Work out the finished part from the listing and answer in its coordinate system (mm). A direction names the side the tool comes from. Give positions to 0.01 mm unless a question says otherwise; leave off trailing zeros. Loops run counter-clockwise (first coordinate to the right, second up) from the corner with the lowest first, then second, coordinate; pieces in that order, holes last.
from build123d import *

# Parameters (mm, degrees)
BOSS_EXTRUDE1_DEPTH      = 12
SKETCH3_R                = 6
CUT_EXTRUDE1_DEPTH       = 12
BOSS_EXTRUDE2_DEPTH      = 10
SKETCH4_3_R              = 25
BOSS_EXTRUDE3_DEPTH      = 44
SKETCH6_R                = 12.5
CUT_EXTRUDE2_DEPTH       = 44
BOSS_EXTRUDE4_REACH      = 152.121
BOSS_EXTRUDE4_END_RADIUS = 25
SKETCH7_W                = 27
SKETCH7_H                = 32
CUT_EXTRUDE3_DEPTH       = 143.520174011
CUT_EXTRUDE3_DEPTH_BACK  = 44
SKETCH8_W                = 3
SKETCH8_H                = 53.670936702
SKETCH9_R                = 6
CUT_EXTRUDE4_DEPTH       = 44
BOSS_EXTRUDE8_DEPTH      = 2.5
BOSS_EXTRUDE9_REACH      = 95.922
BOSS_EXTRUDE9_END_RADIUS = 25
SKETCH11_W               = 5
SKETCH11_H               = 34


with BuildPart() as part:
    # Sketch1 → Boss-Extrude1 (new body)
    with BuildSketch(Plane.XY):
        with BuildLine():
            Line((25, -31.5), (-25, -31.5))
            ThreePointArc((-25, -31.5), (-42.67766953, -24.17766953), (-50, -6.5))
            Line((-50, -6.5), (-50, 31.5))
            Line((-50, 31.5), (50, 31.5))
            Line((50, 31.5), (50, -6.5))
            ThreePointArc((50, -6.5), (42.67766953, -24.17766953), (25, -31.5))
        make_face()
    extrude(amount=BOSS_EXTRUDE1_DEPTH)

    # Sketch3 → Cut-Extrude1 (cut)
    with BuildSketch(Plane.XY.offset(12)):
        with Locations((-25, -6.5)):
            Circle(SKETCH3_R)
        with Locations((25, -6.5)):
            Circle(SKETCH3_R)
    extrude(amount=-CUT_EXTRUDE1_DEPTH, mode=Mode.SUBTRACT)

    # Sketch4 → Boss-Extrude2 (add)
    with BuildSketch(Plane(origin=(0, 31.5, 0), x_dir=(1, 0, 0), z_dir=(0, 1, 0))):
        with BuildLine():
            Line((-50, 0), (50, 0))
            Line((50, 0), (23.906779363, 85.312038053))
            ThreePointArc((23.906779363, 85.312038053), (0, 103), (-23.906779363, 85.312038053))
            Line((-23.906779363, 85.312038053), (-50, 0))
        make_face()
    extrude(amount=-BOSS_EXTRUDE2_DEPTH)

    # Sketch4<3> → Boss-Extrude3 (add)
    with BuildSketch(Plane(origin=(0, 31.5, 0), x_dir=(1, 0, 0), z_dir=(0, 1, 0))):
        with Locations(Location((0, 78, 0), (0, 0, 180))):
            Circle(SKETCH4_3_R)
    extrude(amount=-BOSS_EXTRUDE3_DEPTH)

    # Sketch6 → Cut-Extrude2 (cut)
    with BuildSketch(Plane.XZ.offset(12.5)):
        with Locations((0, -78)):
            Circle(SKETCH6_R)
    extrude(amount=-CUT_EXTRUDE2_DEPTH, mode=Mode.SUBTRACT)

    # Boss-Extrude4: up to this cylinder (the profile starts outside it)
    boss_extrude4_end = Plane(origin=(0, 9.5, -78), z_dir=(0, 1, 0)) * Cylinder(BOSS_EXTRUDE4_END_RADIUS, 355.242, mode=Mode.PRIVATE)
    # Sketch7 → Boss-Extrude4 (add, up to the surface)
    with BuildSketch(Plane(origin=(0, 0, -126), x_dir=(-1, 0, 0), z_dir=(0, 0, -1)), mode=Mode.PRIVATE) as boss_extrude4_sk1:
        with Locations((0, 9.5)):
            Rectangle(SKETCH7_W, SKETCH7_H)
    boss_extrude4_tool1 = extrude(boss_extrude4_sk1.sketch, amount=-BOSS_EXTRUDE4_REACH, mode=Mode.PRIVATE) - boss_extrude4_end
    add(boss_extrude4_tool1.solids().sort_by_distance((0, 9.5, -126))[0])

    # Sketch8 → Cut-Extrude3 (cut, two sides: drawn at the far end of the back side and taken through both)
    with BuildSketch(Plane.XZ.offset(12.5).offset(-CUT_EXTRUDE3_DEPTH_BACK)):
        with Locations((0, -99.480094591)):
            Rectangle(SKETCH8_W, SKETCH8_H)
    extrude(amount=CUT_EXTRUDE3_DEPTH + CUT_EXTRUDE3_DEPTH_BACK, mode=Mode.SUBTRACT)

    # Sketch9 → Cut-Extrude4 (cut)
    with BuildSketch(Plane.ZY.offset(13.5)):
        with Locations(Location((-112.874414164, 9.5, 0), (0, 0, 270))):
            Circle(SKETCH9_R)
    extrude(amount=-CUT_EXTRUDE4_DEPTH, mode=Mode.SUBTRACT)



with BuildPart() as body_2:
    # Sketch10 → Boss-Extrude8 (new, symmetric)
    with BuildSketch(Plane(origin=(0, 0, 0), x_dir=(0, 0, -1), z_dir=(1, 0, 0))):
        Polygon((53, -12.5), (0, -31.5), (0, 21.5), (53, 21.5), align=None)
    extrude(amount=BOSS_EXTRUDE8_DEPTH, both=True)


with BuildPart() as part_1:
    add(part.part)

    add(body_2.part)  # Boss-Extrude9 merges body 2
    # Boss-Extrude9: up to this cylinder (the profile starts outside it)
    boss_extrude9_end = Plane(origin=(0, 4.5, -78), z_dir=(0, 1, 0)) * Cylinder(BOSS_EXTRUDE9_END_RADIUS, 242.844, mode=Mode.PRIVATE)
    # Sketch11 → Boss-Extrude9 (add, up to the surface)
    with BuildSketch(Plane(origin=(0, 0, -53), x_dir=(-1, 0, 0), z_dir=(0, 0, -1)), mode=Mode.PRIVATE) as boss_extrude9_sk1:
        with Locations((0, 4.5)):
            Rectangle(SKETCH11_W, SKETCH11_H)
    boss_extrude9_tool1 = extrude(boss_extrude9_sk1.sketch, amount=BOSS_EXTRUDE9_REACH, mode=Mode.PRIVATE) - boss_extrude9_end
    add(boss_extrude9_tool1.solids().sort_by_distance((0, 4.5, -53))[0])
    add(boss_extrude9_tool1.solids().sort_by_distance((0, 4.5, -53))[1])


solid = part_1.part
Item 1: Find section C-C, the plane y = 18.5. Write down the section's boundary in (x, z), plus the area to 3 significant figures.
Item 2: For faces 1 (the face through (1.5, 10, -104)), 2 (the face through (21, 21.5, -34)), 3 (the face through (13.5, 9.3, -106.7)), determine the directions among +Z, -Z, +X, -X, +Y, -Y from which every point of the face is accessible in a straight line to the end or side of a thin tool.
Item 3: Consider line 1 (X direction, y = 0, z = -108.5); line 2 (Y direction, x = 24.5, z = 5); line 3 (Z direction, x = -3, y = 2.5). Determine where each line is inside the solid, lowest interval first.
Item 4: Find section D-D, the plane x = 0. Write down the section's boundary in (y, z).
Item 5: Find section B-B, the plane x = 21. Write down the section's boundary in (y, z).
Item 6: Find section A-A, the plane y = 9.5. Write down the section's boundary in (x, z).
Item 7: Flat-ended cylindrical pins translate along their axes: pin 1 Ø10.5 at (y, z) = (2.5, -101) entering from +X; pin 2 Ø3.5 at (x, z) = (5, -110) entering from -Y; pin 3 Ø9.5 at (x, z) = (8.5, -117) entering from +Y. Find the tip coordinate at first contact, or state that the pin passes through.
Item 8: Determine the mould class of faces 4 (the face through (1, 0, 12)), 5 (the face through (50, 13, 6)), 6 (the face through (-1.5, 10, -104)) for opening direction X: released by +X, released by -X, zero draft, split by the parting line, or undercut.
Ans:
1. outline: (-50, 0) - (-2.5, 0) - (-2.5, -53.13) arc R25 ccw to (-13.5, -99.04) - (-13.5, -126) - (-1.5, -126) - (-1.5, -90.41) arc R12.5 cw (long way) to (1.5, -90.41) - (1.5, -126) - (13.5, -126) - (13.5, -99.04) arc R25 ccw to (2.5, -53.13) - (2.5, 0) - (50, 0) - (50, 12) - (-50, 12) - close
1. area: 3,490 mm2
2. face 1: -Z, +Y, -Y
2. face 2: +X, -Y
2. face 3: -Z, +X, +Y, -Y
3. line 1: x = -13.5 to -1.5, 1.5 to 13.5
3. line 2: y = -31.5 to -12.48, -0.52 to 31.5
3. line 3: z = -126 to -90.13, -65.87 to -53.18, 0 to 12
4. outline: (-31.5, 0) - (-12.5, -53) - (-12.5, -65.5) - (31.5, -65.5) - (31.5, 12) - (-31.5, 12) - close
5. outline: (-31.5, 0) - (-10.97, 0) - (-10.97, 12) - (-31.5, 12) - close; (-12.5, -91.56) - (31.5, -91.56) - (31.5, 12) - (-2.03, 12) - (-2.03, 0) - (21.5, 0) - (21.5, -64.44) - (-12.5, -64.44) - close
6. outline: (-50, 0) - (-2.5, 0) - (-2.5, -53.13) arc R25 ccw to (-13.5, -99.04) - (-13.5, -106.87) - (-1.5, -106.87) - (-1.5, -90.41) arc R12.5 cw (long way) to (1.5, -90.41) - (1.5, -106.87) - (13.5, -106.87) - (13.5, -99.04) arc R25 ccw to (2.5, -53.13) - (2.5, 0) - (50, 0) - (50, 12) - (-50, 12) - close; (-13.5, -126) - (-1.5, -126) - (-1.5, -118.87) - (-13.5, -118.87) - close; (1.5, -126) - (13.5, -126) - (13.5, -118.87) - (1.5, -118.87) - close
7. pin 1: stops at x = 17.61
7. pin 2: stops at y = -6.5
7. pin 3: stops at y = 25.5
8. face 4: zero draft
8. face 5: released by +X
8. face 6: undercut
